from build123d import *

# Parameters (mm, degrees)
F0_W          = 5.842
F0_H          = 12.7
F0_R          = 3.175
F2_DEPTH      = 3.175
F3_R          = 1.524
F4_DEPTH      = 6.35
F4_DEPTH_BACK = 1.27
F5_R          = 1.524
F7_DEPTH      = 17.78
F6_R          = 1.524
F8_DEPTH      = 10.414
F9_DEPTH      = 56.134


with BuildPart() as f1:
    # F0 (on Front) → F1 (revolve)
    with BuildSketch(Plane.XZ):
        Polygon((5.842, 12.7), (5.842, 0), (66.294, 0), (66.294, 12.7), (56.134, 12.7), (56.134, 10.16), (10.16, 10.16), (10.16, 12.7), align=None)
        with Locations((2.921, 6.35)):
            Rectangle(F0_W, F0_H)
    revolve(axis=Axis((33.147, 0, 0), (-1, 0, 0)))

    # F0 (on Front) → F2 (join, symmetric)
    with BuildSketch(Plane.XZ):
        with Locations((2.921, 6.35)):
            Rectangle(F0_W, F0_H)
        with BuildLine():
            Line((-0.9398, 0), (0, 0))
            Line((0, 0), (0, 12.7))
            Line((0, 12.7), (5.842, 12.7))
            Line((5.842, 12.7), (5.842, 15.24))
            Line((5.842, 15.24), (-0.508, 15.24))
            Line((-0.508, 15.24), (-10.8806298187, 3.8475430269))
            ThreePointArc((-10.8806298187, 3.8475430269), (-4.5919612295, 5.3297205562), (-0.9398, 0))
        make_face()
        with BuildLine():
            Line((5.842, 0), (0, 0))
            Line((0, 0), (-0.9398, 0))
            ThreePointArc((-0.9398, 0), (-3.1957909266, -4.5493385486), (-8.1826630726, -5.5069827884))
            Line((-8.1826630726, -5.5069827884), (5.842, -9.398))
            Line((5.842, -9.398), (5.842, 0))
        make_face()
        with BuildLine():
            ThreePointArc((-8.1826630726, -5.5069827884), (-3.1957909266, -4.5493385486), (-0.9398, 0))
            ThreePointArc((-0.9398, 0), (-4.5919612295, 5.3297205562), (-10.8806298187, 3.8475430269))
            ThreePointArc((-10.8806298187, 3.8475430269), (-12.1459778134, -1.5837270034), (-8.1826630726, -5.5069827884))
        make_face()
        with Locations((-6.6548, 0)):
            Circle(F0_R, mode=Mode.SUBTRACT)
    extrude(amount=F2_DEPTH, both=True)

    # F3 (on face) → F4 (join, two sides)
    with BuildSketch(Plane.YZ.offset(66.294)) as f4_sk:
        with BuildLine():
            ThreePointArc((-5.08, 0), (0, -5.08), (5.08, 0))
            ThreePointArc((5.08, 0), (0, 5.08), (-5.08, 0))
        make_face()
        Circle(F3_R, mode=Mode.SUBTRACT)
        with BuildLine():
            ThreePointArc((-5.08, 0), (0, 5.08), (5.08, 0))
            Line((5.08, 0), (5.08, 15.24))
            Line((5.08, 15.24), (-5.08, 15.24))
            Line((-5.08, 15.24), (-5.08, 0))
        make_face()
    extrude(amount=F4_DEPTH)
    extrude(f4_sk.sketch, amount=-F4_DEPTH_BACK)

    # F5 (on face) → F7 (cut)
    with BuildSketch(Plane.XY.offset(15.24)):
        with Locations((68.834, 0)):
            Circle(F5_R)
    extrude(amount=-F7_DEPTH, mode=Mode.SUBTRACT)

    # F6 (on face) → F8 (cut)
    with BuildSketch(Plane.XY.offset(15.24)):
        with Locations((2.667, 0)):
            Circle(F6_R)
    extrude(amount=-F8_DEPTH, mode=Mode.SUBTRACT)

    # F9 (cut, through all): a face of the model
    f9_faces = [f1.faces().sort_by_distance(p)[0] for p in [
        (66.294, 0, 0),
    ]]
    extrude(f9_faces, amount=-F9_DEPTH, mode=Mode.SUBTRACT)


solid = f1.part
Source: CAD feature listing. Evaluate the final solid. Frame: model axes, mm. A direction names the side the tool comes from. Give positions to 0.01 mm unless a question says otherwise; leave off trailing zeros. Write each loop counter-clockwise with the first axis right and the second up, starting at its lowest first coordinate (ties: lowest second). Pieces come first, ordered by that corner, then holes. Notation, with made-up numbers: M 28.25,8 L 55.25,8 A18 ccw 55.25,43 Z; hole C 21,13.5 d10. An arc over 180 degrees is marked long. Return JSON: item names as keys, results as strings. Group by question number.
1) Cut plane C-C, the plane x = 26. Output: boundary loops of the cut face in (y, z).
2) Ray query, L1, parallel to Y at x = 69.95, z = 0; L2, parallel to X at y = -1.75, z = -8.5; L3, parallel to X at y = 0, z = -0.8. Return the intervals inside material, ascending.
3) Cut plane B-B, the plane z = 6.25. Output: boundary loops of the cut face in (x, y) (3 decimals).
4) Set-up query: faces 1 (the face through (66.294, 0, -6)), 2 (the face through (32.825, 10.074, -1.323)), 3 (the face through (10.16, 0, 0)), 4 (the face through (4.12, 0.46, 10.11)). Return all of +Z, -Z, +X, -X, +Y, -Y with unobstructed straight access to the full face (end or side cutting, diameter ignored); none if empty.
5) Cut plane D-D, the plane y = 4. Output: boundary loops of the cut face in (x, z).
6) Draft query along X for faces 5 (the face through (72.644, 0, 5)), 6 (the face through (69, 5.08, 8)), 7 (the face through (10.16, 9, 6)). Return one class per face: released by +X, released by -X, zero draft, split by the parting line, or undercut.
7) Cut plane A-A, the plane y = 0. Give the number of separate pieces and of enclosed holes in the cut face, then the cut area to 3 significant figures.
8) First-contact query: pin 1 Ø1 at (x, z) = (1, -9) entering from -Y; pin 2 Ø4 at (x, z) = (67, 6.5) entering from -Y; pin 3 Ø1 at (y, z) = (-10, -8) entering from +X; pin 4 Ø3.5 at (x, y) = (69, -0.5) entering from +Z. Flat tips, straight axial feed; report the tip coordinate or a pass-through.
Data:
{
 "1": {"outline": "C 0,0 d20.32; hole C 0,0 d3.05"},
 "2": {"L1": "y = -5.08 to -1.52, 1.52 to 5.08", "L2": "x = 0 to 66.29", "L3": "x = -12.31 to -9.73, -3.58 to 10.16"},
 "3": {"outline": "M -8.693,-3.175 L 0,-3.175 L 0,-11.056 L 10.16,-11.056 L 10.16,-8.01 L 56.134,-8.01 L 56.134,-11.056 L 66.294,-11.056 L 66.294,-5.08 L 72.644,-5.08 L 72.644,5.08 L 66.294,5.08 L 66.294,11.056 L 56.134,11.056 L 56.134,8.01 L 10.16,8.01 L 10.16,11.056 L 0,11.056 L 0,3.175 L -8.693,3.175 Z; hole C 2.667,0 d3.048; hole C 68.834,0 d3.048"},
 "4": {"face 1": "-Z, +X", "face 2": "none", "face 3": "+X", "face 4": "+Z"},
 "5": {"outline": "M 0,-12.05 L 10.16,-12.05 L 10.16,-9.34 L 56.13,-9.34 L 56.13,-12.05 L 66.29,-12.05 L 66.29,-3.13 L 72.64,-3.13 L 72.64,15.24 L 65.02,15.24 L 65.02,12.05 L 56.13,12.05 L 56.13,9.34 L 10.16,9.34 L 10.16,12.05 L 0,12.05 Z"},
 "6": {"face 5": "released by +X", "face 6": "zero draft", "face 7": "undercut"},
 "7": {"separate pieces": "2", "enclosed holes": "1", "area": "1,480 mm²"},
 "8": {"pin 1": "stops at y = -9.44", "pin 2": "stops at y = -11.83", "pin 3": "stops at x = 66.29", "pin 4": "stops at z = 15.24"}
}
